Source: three-view drawing plus pictorial views. Frame: mm from the lowest corner of the part. Coordinates: 2 decimals unless noted, no trailing zeros. Loops run counter-clockwise (first coordinate to the right, second up) from the corner with the lowest first, then second, coordinate; pieces in that order, holes last. Notation, with made-up numbers: M 61,32 L 97,32 A30 cw 97,64 Z; hole C 81.25,23.5 d11. An arc over 180 degrees is marked long. Use a Markdown table: item, result. Add a question column.
1. Section B-B on z = 8. Output: boundary loops of the cut face in (x, y), then the cut area to 3 significant figures.
2. Section C-C on x = 4. Output: boundary loops of the cut face in (y, z), then the cut area to 3 significant figures.
3. Section A-A on y = 4. Output: boundary loops of the cut face in (x, z).
4. Draft query along X for the marked faces 1, 2 and 3. Return one class per face: +X half, -X half, draft (parallel to the pull), parting line (faces both ways), or undercut.
5. Pin query (flat end, axial travel): pin 1 (1.5 mm diameter, centred on x = 12, y = 2.5, fed in from +Z); pin 2 (4 mm diameter, centred on y = 5.5, z = 10, fed in from -X). Return the tip coordinate at first contact, or that it passes through.
6. Line query: L1, parallel to Z at x = 4, y = 6; L2, parallel to X at y = 4.25, z = 7.25; L3, parallel to X at y = 1.5, z = 7.75. Output: solid intervals per line, ascending. Write a range as [from, to].
7. Section D-D on x = 12. Output: boundary loops of the cut face in (y, z).
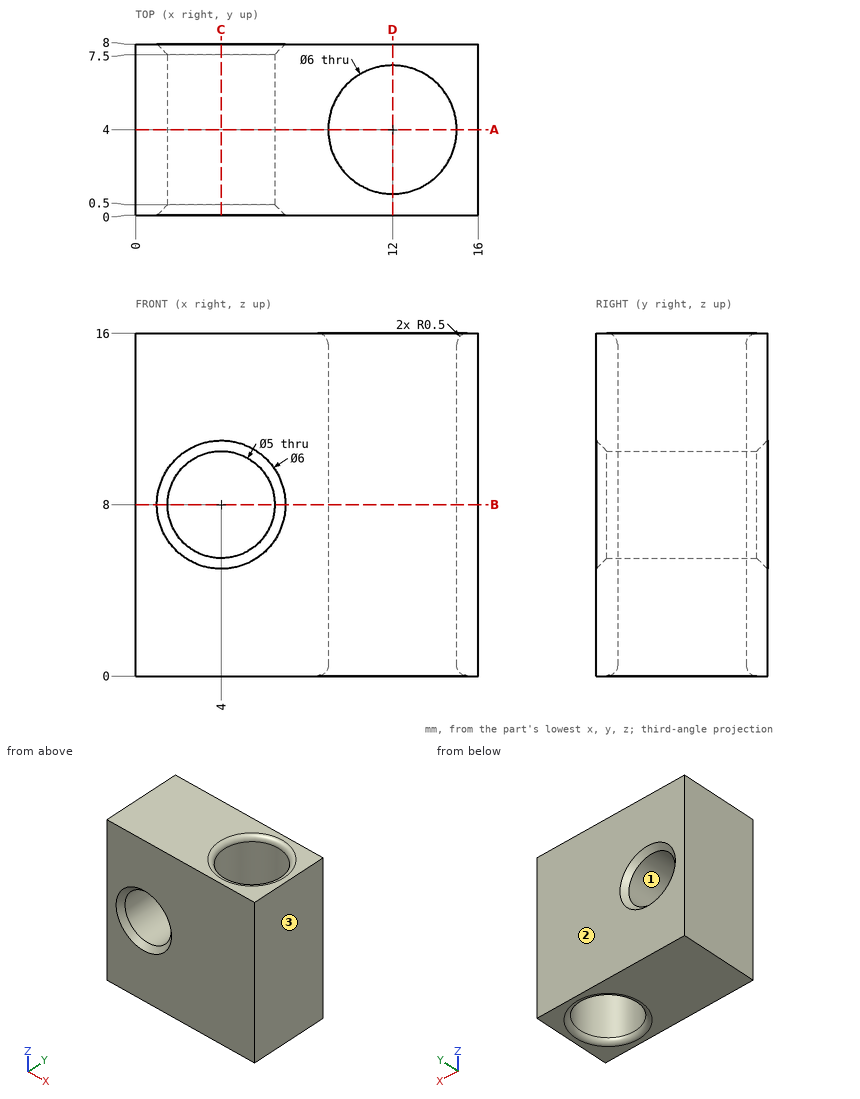
Answers below:
| question | item | result |
|---|---|---|
| 1 | outline | M 0,0 L 1,0 L 1.5,0.5 L 1.5,7.5 L 1,8 L 0,8 Z; M 6.5,0.5 L 7,0 L 16,0 L 16,8 L 7,8 L 6.5,7.5 Z; hole C 12,4 d6 |
| 1 | area | 59.2 mm² |
| 2 | outline | M 0,0 L 8,0 L 8,5 L 7.5,5.5 L 0.5,5.5 L 0,5 Z; M 0,11 L 0.5,10.5 L 7.5,10.5 L 8,11 L 8,16 L 0,16 Z |
| 2 | area | 87.5 mm² |
| 3 | outline | M 0,0 L 8.5,0 A0.5 ccw 9,0.5 L 9,15.5 A0.5 ccw 8.5,16 L 0,16 Z; M 15,0.5 A0.5 ccw 15.5,0 L 16,0 L 16,16 L 15.5,16 A0.5 ccw 15,15.5 Z; hole C 4,8 d5 |
| 4 | face 1 | undercut |
| 4 | face 2 | draft |
| 4 | face 3 | +X half |
| 5 | pin 1 | passes through |
| 5 | pin 2 | stops at x = 0 |
| 6 | L1 | z = [0, 5.5], [10.5, 16] |
| 6 | L2 | x = [0, 1.62], [6.38, 9.01], [14.99, 16] |
| 6 | L3 | x = [0, 1.51], [6.49, 10.34], [13.66, 16] |
| 7 | outline | M 0,0 L 0.5,0 A0.5 ccw 1,0.5 L 1,15.5 A0.5 ccw 0.5,16 L 0,16 Z; M 7,0.5 A0.5 ccw 7.5,0 L 8,0 L 8,16 L 7.5,16 A0.5 ccw 7,15.5 Z |
